The model under review builds one solid part; all positions refer to its coordinate system, in mm. Face numbers are marked on the shaded views. A direction names the side the tool comes from. Give positions to 0.01 mm unless a question says otherwise; leave off trailing zeros. Order: outer loops, then holes, each group sorted by start corner. A loop starts at its lowest first (then second) coordinate and runs counter-clockwise, first axis right, second up. Notation, with made-up numbers: (15.25, -33) - (48.25, -33) arc R12 ccw to (48.25, -11) - close; hole circle Ø11 at (54.5, -6.5). An arc over 180 degrees is marked (long way). Put each result on its own line as item: value.
```python
from build123d import *

# Parameters (mm, degrees)
SKETCH_W        = 59
SKETCH_H        = 53
PAD_DEPTH       = 10
SKETCH001_W     = 55
SKETCH001_H     = 49
POCKET_DEPTH    = 7
SKETCH002_R     = 1.15
HOLE_DEPTH      = 25
SKETCH003_W     = 10
SKETCH003_H     = 3.3
SKETCH003_W_2   = 16.7
SKETCH003_H_2   = 2.3
POCKET001_DEPTH = 5


with BuildPart() as part:
    # Sketch → Pad (new body)
    with BuildSketch(Plane.XY):
        with Locations((29.5, 26.5)):
            Rectangle(SKETCH_W, SKETCH_H)
    extrude(amount=PAD_DEPTH)

    # Sketch001 (on Face6 of Pad) → Pocket (cut)
    with BuildSketch(Plane.XY.offset(10)):
        with Locations((29.5, 26.5)):
            Rectangle(SKETCH001_W, SKETCH001_H)
    extrude(amount=-POCKET_DEPTH, mode=Mode.SUBTRACT)

    # Sketch002 (on Face11 of Pocket) → Hole (cut)
    with BuildSketch(Plane.XY.offset(3)):
        with Locations((5.69, 39.5)):
            Circle(SKETCH002_R)
        with Locations((34.5, 5.7)):
            Circle(SKETCH002_R)
        with Locations((5.69, 5.7)):
            Circle(SKETCH002_R)
        with Locations((51.5, 39.5)):
            Circle(SKETCH002_R)
    extrude(amount=-HOLE_DEPTH, mode=Mode.SUBTRACT)

    # Sketch003 (on Face1 of Hole) → Pocket001 (cut)
    with BuildSketch(Plane.XZ):
        with Locations((26.5, 6.35)):
            Rectangle(SKETCH003_W, SKETCH003_H)
        with Locations((47.65, 5.85)):
            Rectangle(SKETCH003_W_2, SKETCH003_H_2)
    extrude(amount=-POCKET001_DEPTH, mode=Mode.SUBTRACT)


solid = part.part
```
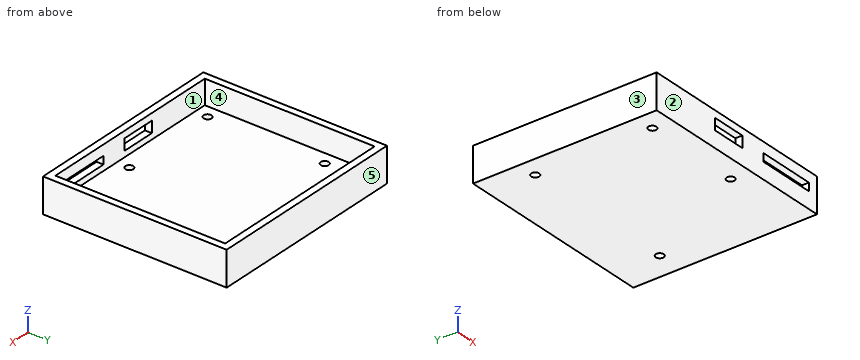
(1) Clearance check with a flat-ended pin moving along its axis: pin 1 Ø3 at (x, y) = (31, 23) entering from +Z. State where the tip first meets the part, or that it passes through.
The answers:
pin 1: z = 3
(2) Wall thickness on L1, parallel to Y at x = 5.69, z = 1.5; L2, parallel to Y at x = 4, z = 8.5; L3, parallel to Y at x = 34.5, z = 1.25: over which ranges is each line inside the solid? List them lowest first.
The answers:
L1: 0 to 4.55, 6.85 to 38.35, 40.65 to 53
L2: 0 to 2, 51 to 53
L3: 0 to 4.55, 6.85 to 53
(3) Take a section at C-C, the plane x = 51.5. Write out the cut boundary in (y, z).
The answers:
outline: (0, 0) - (38.35, 0) - (38.35, 3) - (2, 3) - (2, 4.7) - (0, 4.7) - close; (0, 7) - (2, 7) - (2, 10) - (0, 10) - close; (40.65, 0) - (53, 0) - (53, 10) - (51, 10) - (51, 3) - (40.65, 3) - close
(4) Take a section at B-B, the plane y = 39.5. Write out the cut boundary in (x, z), then the cut area to 3 significant figures.
The answers:
outline: (0, 0) - (4.54, 0) - (4.54, 3) - (2, 3) - (2, 10) - (0, 10) - close; (6.84, 0) - (50.35, 0) - (50.35, 3) - (6.84, 3) - close; (52.65, 0) - (59, 0) - (59, 10) - (57, 10) - (57, 3) - (52.65, 3) - close
area: 191 mm^2
(5) Take a section at D-D, the plane x = 25.5. Write out the cut boundary in (y, z), then the cut area to 3 significant figures.
The answers:
outline: (0, 0) - (53, 0) - (53, 10) - (51, 10) - (51, 3) - (2, 3) - (2, 4.7) - (0, 4.7) - close; (0, 8) - (2, 8) - (2, 10) - (0, 10) - close
area: 180 mm^2
(6) The part is to be moulded in two halves that separate along Y. For the marked faces 1, 2 and 3, say which applies: pulls with the +Y half, pulls with the -Y half, needs draft (parallel to the pull), parting line crosses it, or undercut.
The answers:
face 1: undercut
face 2: pulls with the -Y half
face 3: needs draft
(7) For the marked faces 4 and 5, list the 3-axis set-ups (+Z, -Z, +X, -X, +Y, -Y) from which the entire face can be reached by the end or side of a thin tool; tool diameter is ignored.
The answers:
face 4: +Z
face 5: +Z, -Z, +X, -X, +Y
(8) Take a section at A-A, the plane x = 34.5. Write out the cut boundary in (y, z), then the cut area to 3 significant figures.
The answers:
outline: (0, 0) - (4.55, 0) - (4.55, 3) - (2, 3) - (2, 10) - (0, 10) - close; (6.85, 0) - (53, 0) - (53, 10) - (51, 10) - (51, 3) - (6.85, 3) - close
area: 180 mm^2
